from build123d import *

# Parameters (mm, degrees)
F0_R           = 2.2
F0_W           = 3
F0_H           = 34
F0_R_2         = 1.2
F1_DEPTH       = 1.27
F2_D           = 2.4
F2_CSINK_D     = 4.4
F2_CSINK_ANGLE = 90
F3_DEPTH       = 6.2
F5_W           = 34
F5_H           = 3
F6_DEPTH       = 3
F4_W           = 34
F4_H           = 3
F7_DEPTH       = 3


with BuildPart() as f1:
    # F0 (on Top) → F1 (new body)
    with BuildSketch(Plane.XY):
        with BuildLine():
            Line((-22.6304123436, -30.6505662125), (-22.6304123436, -46.5069715967))
            Line((-22.6304123436, -46.5069715967), (20.3084139398, -46.5069715967))
            Line((20.3084139398, -46.5069715967), (20.3084139398, -30.6505662125))
            Line((20.3084139398, -30.6505662125), (52.2557814969, -30.6505662125))
            Line((52.2557814969, -30.6505662125), (52.2557814969, -10.3231005183))
            ThreePointArc((52.2557814969, -10.3231005183), (51.4252585036, -8.3180406439), (49.4201986292, -7.4875176505))
            Line((49.4201986292, -7.4875176505), (33.2168278796, -7.4875176505))
            ThreePointArc((33.2168278796, -7.4875176505), (28.347396756, -5.4705332381), (26.3304123436, -0.6011021145))
            Line((26.3304123436, -0.6011021145), (26.3304123436, 15.9340094723))
            ThreePointArc((26.3304123436, 15.9340094723), (0, 42.2644218159), (-26.3304123436, 15.9340094723))
            Line((-26.3304123436, 15.9340094723), (-26.3304123436, -0.6011021145))
            ThreePointArc((-26.3304123436, -0.6011021145), (-28.347396756, -5.4705332381), (-33.2168278796, -7.4875176505))
            Line((-33.2168278796, -7.4875176505), (-49.4201986292, -7.4875176505))
            ThreePointArc((-49.4201986292, -7.4875176505), (-51.4252585036, -8.3180406439), (-52.2557814969, -10.3231005183))
            Line((-52.2557814969, -10.3231005183), (-52.2557814969, -30.6505662125))
            Line((-52.2557814969, -30.6505662125), (-22.6304123436, -30.6505662125))
        make_face()
        with Locations((-49.7557814969, -26.6505662125)):
            Circle(F0_R, mode=Mode.SUBTRACT)
        with Locations((49.7557814969, -26.6505662125)):
            Circle(F0_R, mode=Mode.SUBTRACT)
        Polygon((20.7, 8.3494337875), (-20.7, 8.3494337875), (-20.7, -25.6505662125), (-23.7, -25.6505662125), (-23.7, 8.3494337875), (-23.7, 11.3494337875), (23.7, 11.3494337875), (23.7, 8.3494337875), (23.7, -25.6505662125), (20.7, -25.6505662125), align=None, mode=Mode.SUBTRACT)
        with Locations((-23.8304123436, 15.9340094723)):
            Circle(F0_R, mode=Mode.SUBTRACT)
        with Locations((23.8304123436, 15.9340094723)):
            Circle(F0_R, mode=Mode.SUBTRACT)
        Polygon((-23.7, 8.3494337875), (-20.7, 8.3494337875), (20.7, 8.3494337875), (23.7, 8.3494337875), (23.7, 11.3494337875), (-23.7, 11.3494337875), align=None)
        with Locations((-22.2, -8.6505662125)):
            Rectangle(F0_W, F0_H)
        with Locations((22.2, -8.6505662125)):
            Rectangle(F0_W, F0_H)
        with Locations((-23.8304123436, 15.9340094723)):
            Circle(F0_R)
        with Locations((-23.8304123436, 15.9340094723)):
            Circle(F0_R_2, mode=Mode.SUBTRACT)
        with Locations((23.8304123436, 15.9340094723)):
            Circle(F0_R)
        with Locations((23.8304123436, 15.9340094723)):
            Circle(F0_R_2, mode=Mode.SUBTRACT)
        with Locations((49.7557814969, -26.6505662125)):
            Circle(F0_R)
        with Locations((49.7557814969, -26.6505662125)):
            Circle(F0_R_2, mode=Mode.SUBTRACT)
        with Locations((-49.7557814969, -26.6505662125)):
            Circle(F0_R)
        with Locations((-49.7557814969, -26.6505662125)):
            Circle(F0_R_2, mode=Mode.SUBTRACT)
        with Locations((-49.7557814969, -26.6505662125)):
            Circle(F0_R_2)
        with Locations((-23.8304123436, 15.9340094723)):
            Circle(F0_R_2)
        with Locations((23.8304123436, 15.9340094723)):
            Circle(F0_R_2)
        with Locations((49.7557814969, -26.6505662125)):
            Circle(F0_R_2)
    extrude(amount=F1_DEPTH)

    # F2 (through all)
    with Locations(Plane(origin=(0, 0, 0), x_dir=(1, 0, 0), z_dir=(0, 0, -1))):
        with Locations((-49.7557814969, 26.6505662125), (49.7557814969, 26.6505662125), (-23.8304123436, -15.9340094723), (23.8304123436, -15.9340094723)):
            CounterSinkHole(F2_D / 2, F2_CSINK_D / 2, counter_sink_angle=F2_CSINK_ANGLE)

    # F0 (on Top) → F3 (join)
    with BuildSketch(Plane.XY):
        with Locations((-22.2, -8.6505662125)):
            Rectangle(F0_W, F0_H)
        Polygon((-23.7, 8.3494337875), (-20.7, 8.3494337875), (20.7, 8.3494337875), (23.7, 8.3494337875), (23.7, 11.3494337875), (-23.7, 11.3494337875), align=None)
        with Locations((22.2, -8.6505662125)):
            Rectangle(F0_W, F0_H)
    extrude(amount=-F3_DEPTH)

    # F5 (on face) → F6 (join)
    with BuildSketch(Plane(origin=(20.7, 0, 0), x_dir=(0, -1, 0), z_dir=(-1, 0, 0))):
        with Locations((8.6505662125, -4.7)):
            Rectangle(F5_W, F5_H)
    extrude(amount=F6_DEPTH)

    # F4 (on face) → F7 (join)
    with BuildSketch(Plane.YZ.offset(-20.7)):
        with Locations((-8.6505662125, -4.7)):
            Rectangle(F4_W, F4_H)
    extrude(amount=F7_DEPTH)


solid = f1.part
Geometry check sheet. Reference: the model listing, model coordinates, mm. A direction names the side the tool comes from. Give positions to 0.01 mm unless a question says otherwise; leave off trailing zeros. Loops run counter-clockwise (first coordinate to the right, second up) from the corner with the lowest first, then second, coordinate; pieces in that order, holes last. Notation, with made-up numbers: M 39,21 L 95,21 A16 cw 95,47 Z; hole C 66,3 d2. An arc over 180 degrees is marked long. Answer as a JSON object with one key per item and string values. Group by question number.
Item 1: Gauge pin test, flat ends, axial feed: pin 1 (3.5 mm diameter, centred on y = -11, z = -5, fed in from -X); pin 2 (1.9 mm diameter, centred on x = -0.5, z = -3, fed in from -Y); pin 3 (1.5 mm diameter, centred on y = 8, z = 0, fed in from -X); pin 4 (3 mm diameter, centred on x = 49.76, y = -26.65, fed in from +Z). Record the tip position at first contact, or that the pin passes through.
Item 2: Sectioned sample at B-B on x = 0. Record the boundary of the cut face in (y, z), plus the area to 3 significant figures.
Item 3: Sectioned sample at C-C on y = -9. Record the boundary of the cut face in (x, z), plus the area to 3 significant figures.
Item 4: Material ranges on L1, parallel to X at y = 2, z = -1.75; L2, parallel to Z at x = -20.5, y = 3.5; L3, parallel to X at y = -19, z = -5.25, recorded low to high.
Item 5: Access from +Z, -Z, +X, -X, +Y, -Y to the whole of each face (thin tool, end or side, straight path). Record for faces 5 (the flat face through (-21, -25.651, -4)), 6 (the cylindrical face through (28.4, -5.52, 0.63)), 7 (the flat face through (19, -8, -3.2)).
Item 6: Sectioned sample at D-D on x = 13. Record the boundary of the cut face in (y, z).
Item 7: Mould release check, pull along X, two halves, no side actions. Record for faces 1 (the flat face through (0, 11.349, -3)), 2 (the flat face through (-17.7, -9, -5)), 3 (the cylindrical face through (0.58, 42.26, 0.63)), 4 (the flat face through (20.7, -9, -2)): pulls with the +X half, pulls with the -X half, needs draft (parallel to the pull), parting line crosses it, or undercut.
Item 8: Sectioned sample at A-A on y = -19. Record the boundary of the cut face in (x, z), plus the area to 3 significant figures.
Findings below:
{
 "1": {"pin 1": "x = -23.7", "pin 2": "y = 8.35", "pin 3": "x = -26.33", "pin 4": "z = 1.27"},
 "2": {"outline": "M -46.51,0 L 8.35,0 L 8.35,-6.2 L 11.35,-6.2 L 11.35,0 L 42.26,0 L 42.26,1.27 L -46.51,1.27 Z", "area": "131 mm2"},
 "3": {"outline": "M -51.93,0 L -23.7,0 L -23.7,-6.2 L -17.7,-6.2 L -17.7,-3.2 L -20.7,-3.2 L -20.7,0 L 20.7,0 L 20.7,-3.2 L 17.7,-3.2 L 17.7,-6.2 L 23.7,-6.2 L 23.7,0 L 51.93,0 L 51.93,1.27 L -51.93,1.27 Z", "area": "187 mm2"},
 "4": {"L1": "-23.7 to -20.7, 20.7 to 23.7", "L2": "-6.2 to -3.2, 0 to 1.27", "L3": "-23.7 to -17.7, 17.7 to 23.7"},
 "5": {"face 5": "-Z, +X, -X, -Y", "face 6": "+Z, -Z, +X, +Y", "face 7": "-Y"},
 "6": {"outline": "M -46.51,0 L 8.35,0 L 8.35,-6.2 L 11.35,-6.2 L 11.35,0 L 38.83,0 L 38.83,1.27 L -46.51,1.27 Z"},
 "7": {"face 1": "needs draft", "face 2": "undercut", "face 3": "parting line crosses it", "face 4": "undercut"},
 "8": {"outline": "M -52.26,0 L -23.7,0 L -23.7,-6.2 L -17.7,-6.2 L -17.7,-3.2 L -20.7,-3.2 L -20.7,0 L 20.7,0 L 20.7,-3.2 L 17.7,-3.2 L 17.7,-6.2 L 23.7,-6.2 L 23.7,0 L 52.26,0 L 52.26,1.27 L -52.26,1.27 Z", "area": "188 mm2"}
}
